Check sheet for the modelled part. Datum: model origin and axes. Units: mm. A direction names the side the tool comes from. Coordinates: 2 decimals unless noted, no trailing zeros. Loops run counter-clockwise (first coordinate to the right, second up) from the corner with the lowest first, then second, coordinate; pieces in that order, holes last. Notation, with made-up numbers: (-12.75, 22) - (42.25, 22) arc R10 ccw to (42.25, 39) - close; hole circle Ø9 at (-36.75, -28). An arc over 180 degrees is marked (long way). Write each question's results on one line, items separated by ' | '. Start each with the question number.
1. Gauge pin test, flat ends, axial feed: P1, Ø12, axis at y = 54.5, z = -42, coming from the -X side; P2, Ø5, axis at x = 17, z = -17, coming from the +Y side; P3, Ø12, axis at x = 17, z = -26, coming from the +Y side; P4, Ø1, axis at y = 17.5, z = -28, coming from the +X side. Record the tip position at first contact, or that the pin passes through.
2. Tool access check on faces 4 (the face through (53, 7, -29)), 5 (the face through (37, 75, -37)). Record the directions out of +Z, -Z, +X, -X, +Y, -Y that give a thin tool (end or side, any length) a straight path to the whole face; none if there is none.
3. Cross-section at D-D (z = -37). Record the cut outline in (x, y).
4. Draft check along X on faces 1 (the face through (0.9, 3.45, -73.14)), 2 (the face through (73.14, 3.45, -73.1)), 3 (the face through (18.201, 3.549, -60.815)). Enter one of: released by +X, released by -X, zero draft, split by the parting line, or undercut.
5. Cross-section at C-C (x = 37). Record the cut outline in (y, z).
6. Thickness scan on line 1 (X direction, y = 5, z = -57); line 2 (Y direction, x = 21.5, z = -60); line 3 (X direction, y = 48, z = -37). Record the ranges inside material, lowest first. Write a range as [from, to].
7. Cross-section at B-B (z = -17). Record the cut outline in (x, y).
8. Cross-section at A-A (x = 57). Record the cut outline in (y, z).
```python
from build123d import *

# Parameters (mm, degrees)
BOSS_EXTRUDE1_DEPTH = 7
SKETCH2_R           = 15
BOSS_EXTRUDE2_DEPTH = 68
FILLET1_R           = 2
SKETCH3_R           = 4
CUT_EXTRUDE1_DEPTH  = 10


with BuildPart() as part:
    # Sketch1 → Boss-Extrude1 (new body)
    with BuildSketch(Plane(origin=(0, 0, 0), x_dir=(1, 0, 0), z_dir=(0, 1, 0))):
        with BuildLine():
            Line((3, 0), (71, 0))
            ThreePointArc((71, 0), (73.121320344, 0.878679656), (74, 3))
            Line((74, 3), (74, 71))
            ThreePointArc((74, 71), (73.121320344, 73.121320344), (71, 74))
            Line((71, 74), (3, 74))
            ThreePointArc((3, 74), (0.878679656, 73.121320344), (0, 71))
            Line((0, 71), (0, 3))
            ThreePointArc((0, 3), (0.878679656, 0.878679656), (3, 0))
        make_face()
    extrude(amount=BOSS_EXTRUDE1_DEPTH)

    # Sketch2 → Boss-Extrude2 (add)
    with BuildSketch(Plane(origin=(0, 7, 0), x_dir=(1, 0, 0), z_dir=(0, 1, 0))):
        with Locations(Location((37, 37, 0), (0, 0, 270))):
            Circle(SKETCH2_R)
    extrude(amount=BOSS_EXTRUDE2_DEPTH)

    # Fillet1
    fillet1_edges = [part.edges().sort_by_distance(p)[0] for p in [
        (37, 7, -52),
    ]]
    fillet(fillet1_edges, radius=FILLET1_R)

    # Sketch3 → Cut-Extrude1 (cut)
    with BuildSketch(Plane(origin=(0, 7, 0), x_dir=(1, 0, 0), z_dir=(0, 1, 0))):
        with Locations(Location((17, 17, 0), (0, 0, 270))):
            Circle(SKETCH3_R)
        with Locations(Location((57, 17, 0), (0, 0, 270))):
            Circle(SKETCH3_R)
    cut_extrude1 = extrude(amount=-CUT_EXTRUDE1_DEPTH, mode=Mode.SUBTRACT)

    # Mirror1: Cut-Extrude1 across plane
    add(cut_extrude1.mirror(Plane.XY.offset(-37)), mode=Mode.SUBTRACT)


solid = part.part
```
Established:
1) P1: x = 22 | P2: through | P3: y = 7.01 | P4: x = 49.36
2) face 4: +Y | face 5: +Z, -Z, +X, -X, +Y
3) outline: (0, 0) - (74, 0) - (74, 7) - (54, 7) arc R2 cw to (52, 9) - (52, 75) - (22, 75) - (22, 9) arc R2 cw to (20, 7) - (0, 7) - close
4) face 1: released by -X | face 2: released by +X | face 3: undercut
5) outline: (0, -74) - (7, -74) - (7, -54) arc R2 cw to (9, -52) - (75, -52) - (75, -22) - (9, -22) arc R2 cw to (7, -20) - (7, 0) - (0, 0) - close
6) line 1: [0, 13], [21, 53], [61, 74] | line 2: [0, 7] | line 3: [22, 52]
7) outline: (0, 0) - (13, 0) - (13, 7) - (0, 7) - close; (21, 0) - (53, 0) - (53, 7) - (21, 7) - close; (61, 0) - (74, 0) - (74, 7) - (61, 7) - close
8) outline: (0, -74) - (7, -74) - (7, -61) - (0, -61) - close; (0, -53) - (7, -53) - (7, -21) - (0, -21) - close; (0, -13) - (7, -13) - (7, 0) - (0, 0) - close
